```python
from build123d import *

# Parameters (mm, degrees)
F6_DEPTH        = 21
F7_SIZE         = 2
F8_SIZE         = 2
F12_DEPTH       = 2.251
F14_D           = 2.5
F14_CSINK_D     = 4
F14_CSINK_ANGLE = 90


# Not quite as in the source:
# - a feature names something its author has since deleted; it is built from what else it names


with BuildPart() as f6:
    # F5 (on Front) → F6 (new body)
    with BuildSketch(Plane.XZ):
        with BuildLine():
            Line((4.75, 0), (4.75, 4.5))
            Line((4.75, 4.5), (-4.75, 4.5))
            Line((-4.75, 4.5), (-4.75, 0))
            Line((-4.75, 0), (-1.75, 0))
            Line((-1.75, 0), (-1.75, 2.25))
            ThreePointArc((-1.75, 2.25), (0, 4), (1.75, 2.25))
            Line((1.75, 2.25), (1.75, 0))
            Line((1.75, 0), (4.75, 0))
        make_face()
        with BuildLine():
            Line((-1.75, 0), (1.75, 0))
            Line((1.75, 0), (1.75, 2.25))
            ThreePointArc((1.75, 2.25), (0, 4), (-1.75, 2.25))
            Line((-1.75, 2.25), (-1.75, 0))
        make_face()
    extrude(amount=-F6_DEPTH)

    # F7
    f7_edges = [f6.edges().sort_by_distance(p)[0] for p in [
        (-4.75, 10.5, 4.5),
        (4.75, 10.5, 4.5),
    ]]
    chamfer(f7_edges, length=F7_SIZE)

    # F8
    f8_edges = [f6.edges().sort_by_distance(p)[0] for p in [
        (0, 21, 4.5),
    ]]
    chamfer(f8_edges, length=F8_SIZE)

    # F10 (on offset) → F11 (revolve, cut)
    with BuildSketch(Plane.XY.offset(2.25)):
        with BuildLine():
            Line((-1.75, 11.75), (-1.75, 0))
            Line((-1.75, 0), (0, 0))
            Line((0, 0), (0, 13.5))
            ThreePointArc((0, 13.5), (-1.2374368671, 12.9874368671), (-1.75, 11.75))
        make_face()
    revolve(axis=Axis((0, 6.75, 2.25), (0, 1, 0)), mode=Mode.SUBTRACT)

    # F10 (on offset) → F12 (cut, through all)
    with BuildSketch(Plane.XY.offset(2.25)):
        with BuildLine():
            Line((-1.75, 11.75), (-1.75, 0))
            Line((-1.75, 0), (0, 0))
            Line((0, 0), (0, 13.5))
            ThreePointArc((0, 13.5), (-1.2374368671, 12.9874368671), (-1.75, 11.75))
        make_face()
        with BuildLine():
            Line((0, 13.5), (0, 0))
            Line((0, 0), (1.75, 0))
            Line((1.75, 0), (1.75, 11.75))
            ThreePointArc((1.75, 11.75), (1.2374368671, 12.9874368671), (0, 13.5))
        make_face()
    extrude(amount=-F12_DEPTH, mode=Mode.SUBTRACT)

    # F14 (through all)
    with Locations(Plane.XY.offset(4.5)):
        with Locations((0, 16)):
            CounterSinkHole(F14_D / 2, F14_CSINK_D / 2, counter_sink_angle=F14_CSINK_ANGLE)


solid = f6.part
```
Work out the finished part from the listing and answer in its coordinate system (mm). A direction names the side the tool comes from. Round coordinates to 2 decimals unless told otherwise and drop trailing zeros. Loops run counter-clockwise (first coordinate to the right, second up) from the corner with the lowest first, then second, coordinate; pieces in that order, holes last.
(1) The part is cut by section B-B, the plane z = 0.7. Give the vertices of the cut face in (x, y), and give its area (3 significant figures).
Computed values:
outline: (-4.75, 0) - (-1.75, 0) - (-1.75, 11.75) arc R1.75 cw to (1.75, 11.75) - (1.75, 0) - (4.75, 0) - (4.75, 21) - (-4.75, 21) - close; hole circle Ø2.5 at (0, 16)
area: 149 mm2
(2) Find the intervals of material crossed by L1, parallel to X at y = 16, z = 2.05; L2, parallel to X at y = 5.25, z = 1.45; L3, parallel to Y at x = 0, z = 1.1, in increasing order.
Computed values:
L1: x = -4.75 to -1.25, 1.25 to 4.75
L2: x = -4.75 to -1.75, 1.75 to 4.75
L3: y = 13.5 to 14.75, 17.25 to 21
(3) This flat-tipped pin is pushed along its axis until it touches: P1, Ø2, axis at x = 0, y = 16, coming from the +Z side. Where does it stop, or does it pass through?
Computed values:
P1: passes through
(4) For faces 4 (the flat face through (0, 9, 4.5)), 5 (the cylindrical face through (0, 6, 4)), determine the directions among +Z, -Z, +X, -X, +Y, -Y from which every point of the face is accessible in a straight line to the end or side of a thin tool.
Computed values:
face 4: +Z, +X, -X, +Y, -Y
face 5: -Z, -Y
(5) The mould has two halves that part along X. Classify faces 1 (the flat face through (4.75, 10, 1)), 2 (the flat face through (0.1, 20, 3.5)), 3 (the flat face through (1.75, 6, 1)): pulls with the +X half, pulls with the -X half, needs draft (parallel to the pull), parting line crosses it, or undercut.
Computed values:
face 1: pulls with the +X half
face 2: needs draft
face 3: undercut
(6) The part is cut by section A-A, the plane y = 16. Give the vertices of the cut face in (x, z), and give its area (3 significant figures).
Computed values:
outline: (-4.75, 0) - (-1.25, 0) - (-1.25, 3.75) - (-2, 4.5) - (-2.75, 4.5) - (-4.75, 2.5) - close; (1.25, 0) - (4.75, 0) - (4.75, 2.5) - (2.75, 4.5) - (2, 4.5) - (1.25, 3.75) - close
area: 26.9 mm2
(7) The part is cut by section C-C, the plane y = 5.25. Give the vertices of the cut face in (x, z).
Computed values:
outline: (-4.75, 0) - (-1.75, 0) - (-1.75, 2.25) arc R1.75 cw to (1.75, 2.25) - (1.75, 0) - (4.75, 0) - (4.75, 2.5) - (2.75, 4.5) - (-2.75, 4.5) - (-4.75, 2.5) - close
(8) The part is cut by section D-D, the plane x = 3.5. Give the vertices of the cut face in (y, z).
Computed values:
outline: (0, 0) - (21, 0) - (21, 2.5) - (19.75, 3.75) - (0, 3.75) - close
